Could you check a few things on this drawing? It's one solid part, dimensions in mm from its lowest x, y, z. A direction names the side the tool comes from. Round coordinates to 2 decimals unless told otherwise and drop trailing zeros. Loops run counter-clockwise (first coordinate to the right, second up) from the corner with the lowest first, then second, coordinate; pieces in that order, holes last. Notation, with made-up numbers: M 14,59 L 51,59 A5 ccw 51,65 Z; hole C 27,22.25 d2. An arc over 180 degrees is marked long. Put each result on its own line as item: value. Start each with the question number.
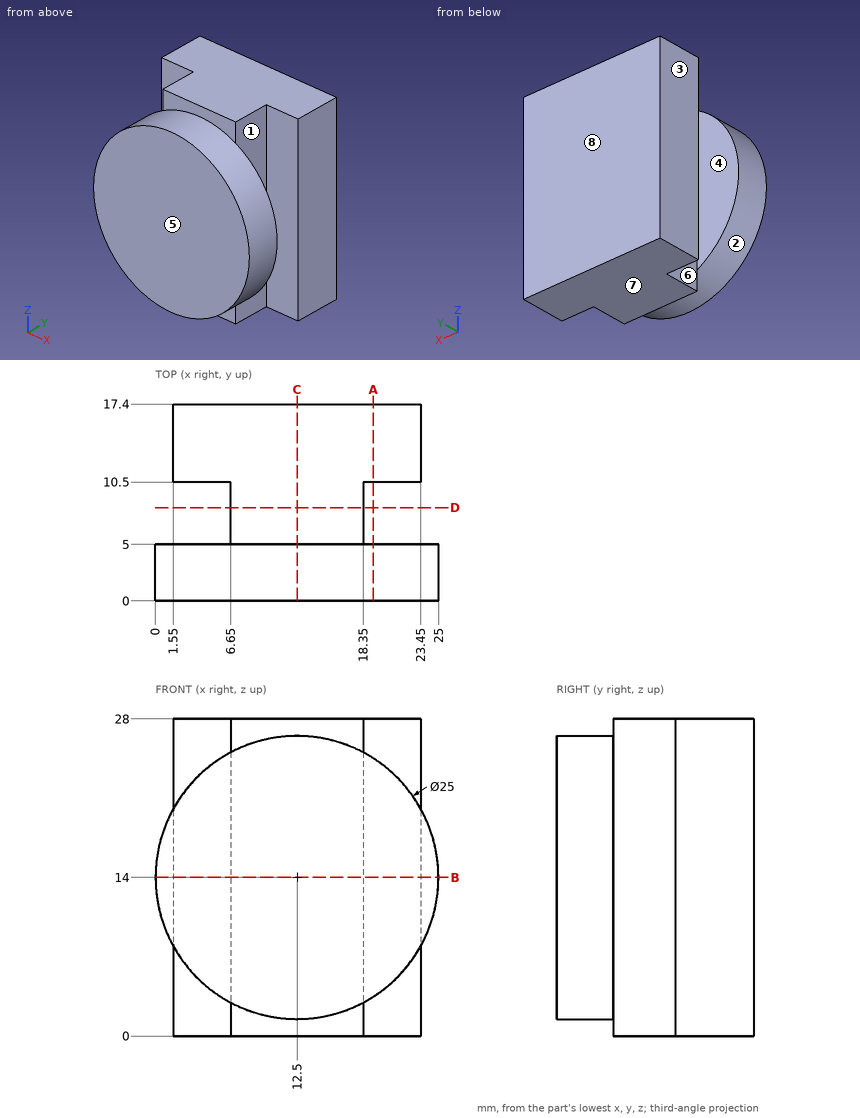
1) Suppose I cut it at D-D (y = 8.25). Write out the boundary of the cut face in (x, z), plus the area to 3 significant figures.
2) If we mould it in two halves opening along Y, with no side actions, what happens to the marked faces 5, 6, 7 and 8? For each: pulls with the +Y half, pulls with the -Y half, needs draft (parallel to the pull), parting line crosses it, or undercut.
3) Suppose I cut it at C-C (x = 12.5). Write out the boundary of the cut face in (y, z), plus the area to 3 significant figures.
4) If I drill on probe 1 along Y at (x, z) = (21, 21); probe 2 along X at (y, z) = (8.5, 2); probe 3 along Y at (x, z) = (21.5, 23.25), over which ranges is the centre line in solid material (lowest first)? Write a range as from..to.
5) Suppose I cut it at A-A (x = 19.25). Write out the boundary of the cut face in (y, z), plus the area to 3 significant figures.
6) Suppose I cut it at B-B (z = 14). Write out the boundary of the cut face in (x, y).
7) On a 3-axis mill with a long thin cutter (end or side, diameter ignored), from which of +Z, -Z, +X, -X, +Y, -Y can I reach the whole of each face in a straight line? I mean the marked faces 1, 2, 3 and 4. Say none if no direction works.
8) I'm going to push flat-ended pins straight in: P1, Ø2, axis at y = 15.5, z = 13.5, coming from the +X side; P2, Ø0.9, axis at x = 10.5, z = 1, coming from the -Y side; P3, Ø6, axis at y = 7.5, z = 20.5, coming from the -X side. Where does each tip first touch, or does it pass through?
Results are:
1. outline: M 6.65,0 L 18.35,0 L 18.35,28 L 6.65,28 Z
1. area: 328 mm²
2. face 5: pulls with the -Y half
2. face 6: undercut
2. face 7: needs draft
2. face 8: pulls with the +Y half
3. outline: M 0,1.5 L 5,1.5 L 5,0 L 17.4,0 L 17.4,28 L 5,28 L 5,26.5 L 0,26.5 Z
3. area: 472 mm²
4. probe 1: 0..5, 10.5..17.4
4. probe 2: 6.65..18.35
4. probe 3: 10.5..17.4
5. outline: M 0,3.48 L 5,3.48 L 5,24.52 L 0,24.52 Z; M 10.5,0 L 17.4,0 L 17.4,28 L 10.5,28 Z
5. area: 298 mm²
6. outline: M 0,0 L 25,0 L 25,5 L 18.35,5 L 18.35,10.5 L 23.45,10.5 L 23.45,17.4 L 1.55,17.4 L 1.55,10.5 L 6.65,10.5 L 6.65,5 L 0,5 Z
7. face 1: +Z, -Z, +X
7. face 2: -Y
7. face 3: +Z, -Z, -X, +Y
7. face 4: +Z, -Z, -X
8. P1: x = 23.45
8. P2: y = 5
8. P3: x = 0.98
